The drawing under review shows one solid part. Ordinate dimensions are in mm from its lowest x, y, z. Coordinates: 2 decimals unless noted, no trailing zeros. Loops run counter-clockwise (first coordinate to the right, second up) from the corner with the lowest first, then second, coordinate; pieces in that order, holes last. Notation, with made-up numbers: (-20.75, -3.75) - (-11.75, -3.75) arc R20 ccw to (-11.75, 14.25) - close; hole circle Ø2 at (-17, 27). An arc over 180 degrees is marked (long way). Answer as a JSON object with one key per item and string values. Group by question number.
Item 1: Clearance check with flat-ended pins moving along their axes: pin 1 (5 mm diameter, centred on x = 25.5, y = 2, fed in from -Z); pin 2 (4 mm diameter, centred on x = 5.08, y = 4.76, fed in from +Z). State where each tip first meets the part, or that it passes through.
Item 2: We need section D-D (z = 46). Give the boundary of the cut face in (x, y) (1 decimal).
Item 3: To check wall thickness, follow line 1 (X direction, y = 4.75, z = 48.5); line 2 (X direction, y = 7, z = 11) (1 decimal); line 3 (Y direction, x = 5, z = 19) (1 decimal). State the ranges of each line that lie inside material, in increasing order.
Item 4: We need section C-C (x = 44). Give the boundary of the cut face in (y, z) (1 decimal).
Item 5: We need section A-A (x = 5.08). Give the boundary of the cut face in (y, z) (1 decimal), then the cut area to 3 significant figures.
Item 6: We need section B-B (y = 5.5). Give the boundary of the cut face in (x, z), then the cut area to 3 significant figures.
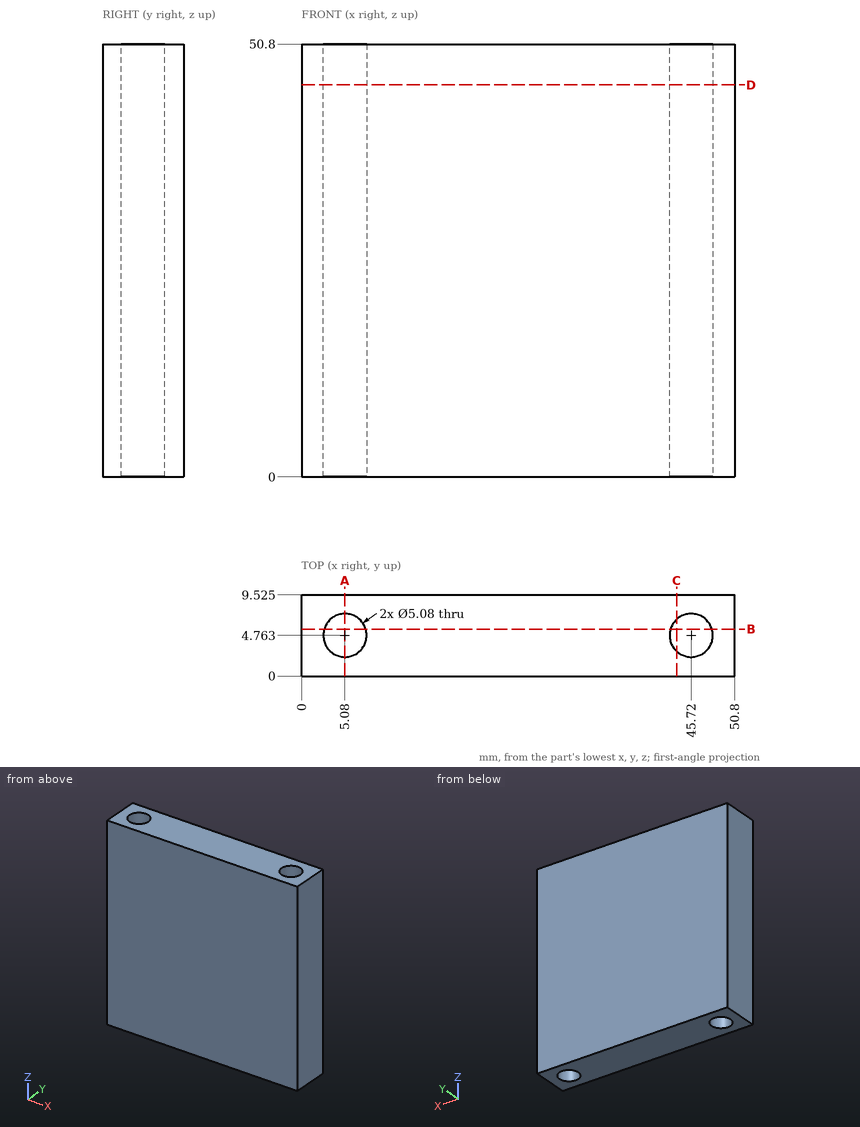
Check sheet entries:
{
 "1": {"pin 1": "stops at z = 0", "pin 2": "passes through"},
 "2": {"outline": "(0, 0) - (50.8, 0) - (50.8, 9.5) - (0, 9.5) - close; hole circle Ø5.1 at (5.1, 4.8); hole circle Ø5.1 at (45.7, 4.8)"},
 "3": {"line 1": "x = 0 to 2.54, 7.62 to 43.18, 48.26 to 50.8", "line 2": "x = 0 to 3.9, 6.3 to 44.5, 46.9 to 50.8", "line 3": "y = 0 to 2.2, 7.3 to 9.5"},
 "4": {"outline": "(0, 0) - (2.9, 0) - (2.9, 50.8) - (0, 50.8) - close; (6.6, 0) - (9.5, 0) - (9.5, 50.8) - (6.6, 50.8) - close"},
 "5": {"outline": "(0, 0) - (2.2, 0) - (2.2, 50.8) - (0, 50.8) - close; (7.3, 0) - (9.5, 0) - (9.5, 50.8) - (7.3, 50.8) - close", "area": "226 mm2"},
 "6": {"outline": "(0, 0) - (2.65, 0) - (2.65, 50.8) - (0, 50.8) - close; (7.51, 0) - (43.29, 0) - (43.29, 50.8) - (7.51, 50.8) - close; (48.15, 0) - (50.8, 0) - (50.8, 50.8) - (48.15, 50.8) - close", "area": "2,090 mm2"}
}
